from build123d import *

# Parameters (mm, degrees)
ESQUISSE1_W        = 225.94062
ESQUISSE1_H        = 163.6522
ESQUISSE1_R        = 1.5
ESQUISSE1_W_2      = 73
ESQUISSE1_H_2      = 142
BOSS_EXTRU_1_DEPTH = 5
CONG_2_R           = 18.3


with BuildPart() as part:
    # Esquisse1 → Boss.-Extru.1 (new body)
    with BuildSketch(Plane(origin=(0, 0, 0), x_dir=(1, 0, 0), z_dir=(0, 1, 0))):
        Rectangle(ESQUISSE1_W, ESQUISSE1_H)
        with Locations(Location((-105.09631, 73.6981, 0), (0, 0, 270))):
            Circle(ESQUISSE1_R, mode=Mode.SUBTRACT)
        with Locations(Location((-35.04311, 76.5429, 0), (0, 0, 270))):
            Circle(ESQUISSE1_R, mode=Mode.SUBTRACT)
        with Locations(Location((-107.63631, 0, 0), (0, 0, 270))):
            Circle(ESQUISSE1_R, mode=Mode.SUBTRACT)
        with Locations(Location((107.63631, 0, 0), (0, 0, 90))):
            Circle(ESQUISSE1_R, mode=Mode.SUBTRACT)
        with Locations(Location((35.04311, 76.5429, 0), (0, 0, 90))):
            Circle(ESQUISSE1_R, mode=Mode.SUBTRACT)
        with Locations(Location((105.09631, 73.6981, 0), (0, 0, 90))):
            Circle(ESQUISSE1_R, mode=Mode.SUBTRACT)
        with Locations(Location((105.09631, -73.6981, 0), (0, 0, 270))):
            Circle(ESQUISSE1_R, mode=Mode.SUBTRACT)
        with Locations(Location((35.04311, -76.5429, 0), (0, 0, 270))):
            Circle(ESQUISSE1_R, mode=Mode.SUBTRACT)
        with Locations(Location((-35.04311, -76.5429, 0), (0, 0, 90))):
            Circle(ESQUISSE1_R, mode=Mode.SUBTRACT)
        with Locations(Location((-105.09631, -73.6981, 0), (0, 0, 90))):
            Circle(ESQUISSE1_R, mode=Mode.SUBTRACT)
        with Locations((-62.47031, 0)):
            Rectangle(ESQUISSE1_W_2, ESQUISSE1_H_2, mode=Mode.SUBTRACT)
        with Locations((20.52969, 0)):
            Rectangle(ESQUISSE1_W_2, ESQUISSE1_H_2, mode=Mode.SUBTRACT)
    extrude(amount=BOSS_EXTRU_1_DEPTH)

    # Congé2
    cong_2_edges = [part.edges().sort_by_distance(p)[0] for p in [
        (-112.97031, 2.5, -81.8261),
        (112.97031, 2.5, -81.8261),
        (112.97031, 2.5, 81.8261),
        (-112.97031, 2.5, 81.8261),
    ]]
    fillet(cong_2_edges, radius=CONG_2_R)


solid = part.part
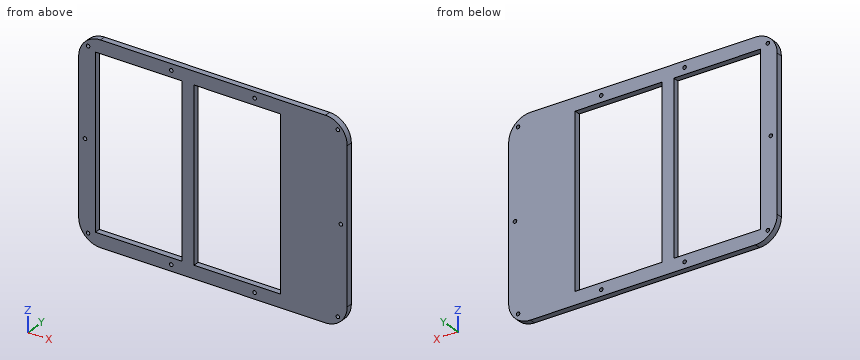
Can you work these out from the model? Positions are in its coordinate system, mm. Give positions to 0.01 mm unless a question says otherwise; leave off trailing zeros. Order: outer loops, then holes, each group sorted by start corner. A loop starts at its lowest first (then second) coordinate and runs counter-clockwise, first axis right, second up. Notation, with made-up numbers: M 12.5,12 L 44.5,12 A9 cw 44.5,27 Z; hole C 11.5,7 d4. An arc over 180 degrees is marked long. Use a Markdown table: item, result. Add a question column.
Item 1: Suppose I cut it at C-C (y = 2.2). Count the separate pieces of the cut face and the enclosed holes in it, then the cut area to 3 significant figures.
Item 2: Will this pin go through, and if not, where does the flat tip stop? pin 1 (2.5 mm diameter, centred on x = -35.04, z = -76.54, fed in from -Y).
Item 3: If I drill on L1, parallel to Z at x = -35, y = 2.05; L2, parallel to X at y = 3.05, z = 64; L3, parallel to X at y = 1.4, z = 64.5, over which ranges is the centre line in solid material (lowest first)? Write a range as [from, to].
Item 4: Suppose I cut it at A-A (x = -64.5). List the corners of the cut face in (y, z) for me.
Item 5: Suppose I cut it at B-B (z = 27). List the corners of the cut face in (x, y) for me, then the cut area to 3 significant figures.
Answer sheet:
| question | item | result |
|---|---|---|
| 1 | separate pieces | 1 |
| 1 | enclosed holes | 12 |
| 1 | area | 15,900 mm² |
| 2 | pin 1 | passes through |
| 3 | L1 | z = [-81.83, -78.04], [-75.04, -71], [71, 75.04], [78.04, 81.83] |
| 3 | L2 | x = [-112.96, -98.97], [-25.97, -15.97], [57.03, 112.96] |
| 3 | L3 | x = [-112.94, -98.97], [-25.97, -15.97], [57.03, 112.94] |
| 4 | outline | M 0,-81.83 L 5,-81.83 L 5,-71 L 0,-71 Z; M 0,71 L 5,71 L 5,81.83 L 0,81.83 Z |
| 5 | outline | M -112.97,0 L -98.97,0 L -98.97,5 L -112.97,5 Z; M -25.97,0 L -15.97,0 L -15.97,5 L -25.97,5 Z; M 57.03,0 L 112.97,0 L 112.97,5 L 57.03,5 Z |
| 5 | area | 400 mm² |
